```python
from build123d import *

# Parameters (mm, degrees)
BOSS_EXTRU_1_DEPTH      = 167.45
ESQUISSE2_W             = 20
ESQUISSE2_H             = 81.618795027
ESQUISSE2_W_2           = 15
ESQUISSE2_W_3           = 3
ESQUISSE2_H_2           = 2
ENL_V_MAT_EXTRU_1_DEPTH = 53.497474683
ESQUISSE3_R             = 3.8
ESQUISSE3_R_2           = 1.725
BOSS_EXTRU_2_DEPTH      = 3
ESQUISSE4_R             = 1.5
BOSS_EXTRU_3_DEPTH      = 3
ESQUISSE5_W             = 3
ESQUISSE5_H             = 45.77
BOSS_EXTRU_4_DEPTH      = 3
CONG_1_R                = 3


with BuildPart() as part:
    # Esquisse1 → Boss.-Extru.1 (new body)
    with BuildSketch(Plane.XY):
        with BuildLine():
            Line((-6.808328014, -1.100662076), (-56.305802697, -50.598136759))
            Line((-56.305802697, -50.598136759), (-54.184482354, -52.719457103))
            Line((-54.184482354, -52.719457103), (-4.687007671, -3.22198242))
            ThreePointArc((-4.687007671, -3.22198242), (-4.036689417, -2.248712373), (-3.808328014, -1.100662076))
            Line((-3.808328014, -1.100662076), (-3.808328014, 98.899337924))
            Line((-3.808328014, 98.899337924), (-6.808328014, 98.899337924))
            Line((-6.808328014, 98.899337924), (-6.808328014, -1.100662076))
        make_face()
    extrude(amount=BOSS_EXTRU_1_DEPTH)

    # Esquisse2 → Enlèv. mat.-Extru.1 (cut, through all)
    with BuildSketch(Plane(origin=(-3.808328014, 0, 0), x_dir=(0, 0, -1), z_dir=(1, 0, 0))):
        with Locations((-150, -11.91005959)):
            Rectangle(ESQUISSE2_W, ESQUISSE2_H)
        with Locations((-7.5, -11.91005959)):
            Rectangle(ESQUISSE2_W_2, ESQUISSE2_H)
        with Locations((-77.5, -11.91005959)):
            Rectangle(ESQUISSE2_W, ESQUISSE2_H)
        with Locations((-165.95, 75.669337924)):
            Rectangle(ESQUISSE2_W_3, ESQUISSE2_H_2)
        with Locations((-1.5, 75.669337924)):
            Rectangle(ESQUISSE2_W_3, ESQUISSE2_H_2)
    extrude(amount=-ENL_V_MAT_EXTRU_1_DEPTH, mode=Mode.SUBTRACT)

    # Esquisse3 → Boss.-Extru.2 (add)
    with BuildSketch(Plane.XY.offset(167.45)):
        with BuildLine():
            Line((-6.808328014, 98.899337924), (-17.923328014, 98.899337924))
            ThreePointArc((-17.923328014, 98.899337924), (-29.038328014, 87.784337924), (-17.923328014, 76.669337924))
            Line((-17.923328014, 76.669337924), (-6.808328014, 76.669337924))
            Line((-6.808328014, 76.669337924), (-6.808328014, 98.899337924))
        make_face()
        with Locations((-17.923328014, 87.784337924)):
            Circle(ESQUISSE3_R, mode=Mode.SUBTRACT)
        with Locations((-25.863328014, 87.453430664)):
            Circle(ESQUISSE3_R_2, mode=Mode.SUBTRACT)
        with Locations((-17.923328014, 95.393430664)):
            Circle(ESQUISSE3_R_2, mode=Mode.SUBTRACT)
        with Locations((-9.983328014, 87.453430664)):
            Circle(ESQUISSE3_R_2, mode=Mode.SUBTRACT)
        with Locations((-17.923328014, 79.513430664)):
            Circle(ESQUISSE3_R_2, mode=Mode.SUBTRACT)
    extrude(amount=-BOSS_EXTRU_2_DEPTH)

    # Esquisse4 → Boss.-Extru.3 (add)
    with BuildSketch(Plane(origin=(0, 0, 0), x_dir=(-1, 0, 0), z_dir=(0, 0, -1))):
        with BuildLine():
            Line((6.808328014, 98.899337924), (17.923328014, 98.899337924))
            ThreePointArc((17.923328014, 98.899337924), (29.038328014, 87.784337924), (17.923328014, 76.669337924))
            Line((17.923328014, 76.669337924), (6.808328014, 76.669337924))
            Line((6.808328014, 76.669337924), (6.808328014, 98.899337924))
        make_face()
        with Locations((17.923328014, 87.784337924)):
            Circle(ESQUISSE4_R, mode=Mode.SUBTRACT)
    extrude(amount=-BOSS_EXTRU_3_DEPTH)

    # Esquisse5 → Boss.-Extru.4 (add)
    with BuildSketch(Plane(origin=(0, 0, 0), x_dir=(-1, 0, 0), z_dir=(0, 0, -1))):
        with Locations((5.308328014, 51.784337924)):
            Rectangle(ESQUISSE5_W, ESQUISSE5_H)
    extrude(amount=BOSS_EXTRU_4_DEPTH)

    # Congé1
    cong_1_edges = [part.edges().sort_by_distance(p)[0] for p in [
        (-3.808328014, 87.784337924, 0),
        (-3.808328014, 87.784337924, 167.45),
    ]]
    fillet(cong_1_edges, radius=CONG_1_R)


solid = part.part
```
Input: part model. Units: mm. Frame: model coordinates. A direction names the side the tool comes from. Give positions to 0.01 mm unless a question says otherwise; leave off trailing zeros. Loops run counter-clockwise (first coordinate to the right, second up) from the corner with the lowest first, then second, coordinate; pieces in that order, holes last.
1) Contact query for flat-ended pins moving along their axis: pin 1 (3.5 mm diameter, centred on x = -8.5, z = 2, fed in from -Y); pin 2 (8 mm diameter, centred on x = -12.5, z = 112.5, fed in from -Y) (3 decimals); pin 3 (2.5 mm diameter, centred on x = -4.5, z = -1, fed in from +Y). Output: stop coordinate, or through.
A:
pin 1: stops at y = 28.9
pin 2: stops at y = -15.035
pin 3: stops at y = 74.67
2) Section query C-C on z = 107. Return the cut outline in (x, y), and give its area (3 significant figures).
A:
outline: (-56.31, -50.6) - (-54.18, -52.72) - (-4.69, -3.22) arc R3 ccw to (-3.81, -1.1) - (-3.81, 98.9) - (-6.81, 98.9) - (-6.81, -1.1) - close
area: 514 mm2
3) Section query D-D on y = 43. Return the cut outline in (x, z), and give its area (3 significant figures).
A:
outline: (-6.81, -3) - (-3.81, -3) - (-3.81, 167.45) - (-6.81, 167.45) - close
area: 511 mm2
4) Line query: L1, parallel to X at y = 47, z = 112.5; L2, parallel to Y at x = -6.5, z = 5; L3, parallel to X at y = -17, z = 92.5. Output: solid intervals per line, ascending.
A:
L1: x = -6.81 to -3.81
L2: y = 28.9 to 98.9
L3: x = -22.71 to -18.47
5) Section query A-A on y = 27. Return the cut outline in (x, z), and give its area (3 significant figures).
A:
outline: (-6.81, 15) - (-3.81, 15) - (-3.81, 67.5) - (-6.81, 67.5) - close; (-6.81, 87.5) - (-3.81, 87.5) - (-3.81, 140) - (-6.81, 140) - close; (-6.81, 160) - (-3.81, 160) - (-3.81, 167.45) - (-6.81, 167.45) - close
area: 337 mm2
6) Reachability of faces 4 (the flat face through (-16, 88, 3)), 5 (the flat face through (-20, -15, 140)), 6 (the flat face through (-31.21, -25.5, 163.67)), 7 (the flat face through (-13, 88, 164.45)), 8 (the flat face through (-16, 88, 0)) from +Z, -Z, +X, -X, +Y, -Y: full face, straight path, thin tool, end or side. Return the list, or none.
A:
face 4: -X, +Y, -Y
face 5: +X, -X, -Y
face 6: +Z, -Z, -X
face 7: -X, +Y
face 8: -Z, +X, -X, +Y, -Y
7) Section query B-B on x = -51. Return the cut outline in (y, z), and give its area (3 significant figures).
A:
outline: (-49.53, 15) - (-45.29, 15) - (-45.29, 67.5) - (-49.53, 67.5) - close; (-49.53, 87.5) - (-45.29, 87.5) - (-45.29, 140) - (-49.53, 140) - close; (-49.53, 160) - (-45.29, 160) - (-45.29, 167.45) - (-49.53, 167.45) - close
area: 477 mm2
8) Mould query, pull axis Y, two halves, no side actions, for faces 1 (the flat face through (-29.782, -28.317, 113.382)), 2 (the cylindrical face through (-15.9, 91, 166)), 3 (the flat face through (-20, -15, 160)). Classes: released by +Y, released by -Y, zero draft, split by the parting line, or undercut.
A:
face 1: released by -Y
face 2: undercut
face 3: zero draft
